```python
from build123d import *

# Parameters (mm, degrees)
SKETCH1_W               = 44
SKETCH1_H               = 20
SKETCH1_R               = 4
SKETCH1_R_2             = 2.55
BOSS_EXTRUDE1_DEPTH     = 7.5
SKETCH2_R               = 2.55
BOSS_EXTRUDE2_DEPTH     = 2.5
SKETCH3_W               = 44
SKETCH3_H               = 5
BOSS_EXTRUDE3_DEPTH     = 10
CUT_EXTRUDE1_DEPTH      = 53.306787322
CUT_EXTRUDE1_DEPTH_BACK = 5


# Read off the part's stored shape, not the designer's step: Sweep1
with BuildPart() as part:
    # Sketch1 → Boss-Extrude1 (new body)
    # profile 1 of 3: a face of its own
    with BuildSketch(Plane(origin=(0, 0, 0), x_dir=(1, 0, 0), z_dir=(0, 1, 0))):
        with BuildLine():
            Line((0, 14), (-6, 14))
            ThreePointArc((-6, 14), (-3.171572875, 12.828427125), (-2, 10))
            ThreePointArc((-2, 10), (-3.171572875, 7.171572875), (-6, 6))
            Line((-6, 6), (0, 6))
            Line((0, 6), (0, 14))
        make_face()
    # profile 2 of 3: a face of its own
    with BuildSketch(Plane(origin=(0, 0, 0), x_dir=(1, 0, 0), z_dir=(0, 1, 0))):
        with Locations((22, 10)):
            Rectangle(SKETCH1_W, SKETCH1_H)
    # profile 3 of 3: a face of its own
    with BuildSketch(Plane(origin=(0, 0, 0), x_dir=(1, 0, 0), z_dir=(0, 1, 0))):
        with Locations((-6, 10)):
            Circle(SKETCH1_R)
        with Locations(Location((-6, 10, 0), (0, 0, 270))):
            Circle(SKETCH1_R_2, mode=Mode.SUBTRACT)
    extrude(amount=BOSS_EXTRUDE1_DEPTH)

    # Sketch2 → Boss-Extrude2 (add)
    # profile 1 of 4: a face of its own
    with BuildSketch(Plane(origin=(0, 7.5, 0), x_dir=(1, 0, 0), z_dir=(0, 1, 0))):
        with BuildLine():
            Line((-6, 6), (0, 6))
            Line((0, 6), (0, 14))
            Line((0, 14), (-6, 14))
            ThreePointArc((-6, 14), (-3.171572875, 12.828427125), (-2, 10))
            ThreePointArc((-2, 10), (-3.171572875, 7.171572875), (-6, 6))
        make_face()
    # profile 2 of 4: a face of its own
    with BuildSketch(Plane(origin=(0, 7.5, 0), x_dir=(1, 0, 0), z_dir=(0, 1, 0))):
        with BuildLine():
            ThreePointArc((-6, 14), (-10, 10), (-6, 6))
            ThreePointArc((-6, 6), (-3.171572875, 7.171572875), (-2, 10))
            ThreePointArc((-2, 10), (-3.171572875, 12.828427125), (-6, 14))
        make_face()
        with Locations(Location((-6, 10, 0), (0, 0, 270))):
            Circle(SKETCH2_R, mode=Mode.SUBTRACT)
    # profile 3 of 4: a face of its own
    with BuildSketch(Plane(origin=(0, 7.5, 0), x_dir=(1, 0, 0), z_dir=(0, 1, 0))):
        with Locations(Location((-6, 10, 0), (0, 0, 270))):
            Circle(SKETCH2_R)
    # profile 4 of 4: a face of its own
    with BuildSketch(Plane(origin=(0, 7.5, 0), x_dir=(1, 0, 0), z_dir=(0, 1, 0))):
        Polygon((0, 0), (44, 0), (44, 20), (0, 20), (0, 14), (0, 6), align=None)
    extrude(amount=BOSS_EXTRUDE2_DEPTH)

    # Sketch3 → Boss-Extrude3 (add)
    with BuildSketch(Plane(origin=(0, 10, 0), x_dir=(1, 0, 0), z_dir=(0, 1, 0))):
        with Locations((22, 2.5)):
            Rectangle(SKETCH3_W, SKETCH3_H)
        with Locations((22, 17.5)):
            Rectangle(SKETCH3_W, SKETCH3_H)
    extrude(amount=BOSS_EXTRUDE3_DEPTH)

    # Sketch4 → Cut-Extrude1 (cut, two sides: drawn at the far end of the back side and taken through both)
    with BuildSketch(Plane(origin=(0, 0, -20), x_dir=(-1, 0, 0), z_dir=(0, 0, -1)).offset(-CUT_EXTRUDE1_DEPTH_BACK)):
        with BuildLine():
            Line((-5, 17.75), (-39, 17.75))
            ThreePointArc((-39, 17.75), (-37.055456352, 16.944543648), (-36.25, 15))
            ThreePointArc((-36.25, 15), (-37.055456352, 13.055456352), (-39, 12.25))
            Line((-39, 12.25), (-5, 12.25))
            ThreePointArc((-5, 12.25), (-7.75, 15), (-5, 17.75))
        make_face()
        with BuildLine():
            ThreePointArc((-36.25, 15), (-37.055456352, 16.944543648), (-39, 17.75))
            Line((-39, 17.75), (-39, 12.25))
            ThreePointArc((-39, 12.25), (-37.055456352, 13.055456352), (-36.25, 15))
        make_face()
        with BuildLine():
            Line((-39, 12.25), (-39, 17.75))
            ThreePointArc((-39, 17.75), (-41.75, 15), (-39, 12.25))
        make_face()
        with BuildLine():
            ThreePointArc((-2.25, 15), (-3.055456352, 16.944543648), (-5, 17.75))
            Line((-5, 17.75), (-5, 12.25))
            ThreePointArc((-5, 12.25), (-3.055456352, 13.055456352), (-2.25, 15))
        make_face()
        with BuildLine():
            Line((-5, 12.25), (-5, 17.75))
            ThreePointArc((-5, 17.75), (-7.75, 15), (-5, 12.25))
        make_face()
    extrude(amount=CUT_EXTRUDE1_DEPTH + CUT_EXTRUDE1_DEPTH_BACK, mode=Mode.SUBTRACT)

    # Sweep1 outline → Sweep1 (revolve)
    with BuildSketch(Plane(origin=(-6, 0, -10), x_dir=(1, 0, 0), z_dir=(0, 0, 1))):
        Polygon((4, 10), (4, 0), (11, 0), (20.5, -5), (38, -5), (38, 0), (20.5, 0), (10.999999705, 10.000000311), align=None)
    revolve(axis=Axis((-6, 0, -10), (0, 1, 0)))


solid = part.part
```
CAD build for the part. Positions are in the model's coordinates, mm. A direction names the side the tool comes from. Round coordinates to 2 decimals unless told otherwise and drop trailing zeros. Write each loop counter-clockwise with the first axis right and the second up, starting at its lowest first coordinate (ties: lowest second). Pieces come first, ordered by that corner, then holes. Notation, with made-up numbers: (72, 76) -> (123, 76) arc R23 ccw to (123, 89) -> close; hole circle Ø8 at (-36, 51.5). An arc over 180 degrees is marked (long way). Answer in a Markdown table with one row per item. Add a question column.
Item 1: Drop flat-ended pins along their axis: pin 1 Ø6 at (x, y) = (15.5, 4) entering from +Z; pin 2 Ø6.5 at (x, z) = (-5.5, -10.5) entering from -Y; pin 3 Ø3 at (x, y) = (15.5, 17) entering from -Z. Give the stop position or say it passes through.
Item 2: Which spindle directions (+Z, -Z, +X, -X, +Y, -Y) get a long thin tool onto all of the face, cutting with end or side? Do faces 4 (the face through (22, 15, -5)), 5 (the face through (-6, 7.5, -10)), 6 (the face through (22, 12.25, -17)), 7 (the face through (22, 20, -18)), 8 (the face through (44, 8, -10)). Say none if no direction does.
Item 3: Saw through at C-C, the plane z = -37.5. Write the cut outline in (x, y).
Item 4: Drill centre lines: line 1 (Z direction, x = 4, y = 11.75); line 2 (Y direction, x = -5, z = -35). Where is each one in solid material? Low to high. Write a range as from..to.
Item 5: Saw through at B-B, the plane y = 1. Write the cut outline in (x, z).
Item 6: Mould opens along X. For faces 1 (the face through (22, 10, -20)), 2 (the face through (41.75, 15.06, -17.46)), 3 (the face through (30.245, -2.465, -21.414)) say: pulls with the +X half, pulls with the -X half, needs draft (parallel to the pull), parting line crosses it, or undercut.
Item 7: Saw through at A-A, the plane x = 29.5. Write the cut outline in (y, z).
Item 8: Saw through at D-D, the plane x = -36.5. Write the cut outline in (y, z).
Findings below:
| question | item | result |
|---|---|---|
| 1 | pin 1 | stops at z = 0 |
| 1 | pin 2 | stops at y = 0 |
| 1 | pin 3 | stops at z = -20 |
| 2 | face 4 | +X, -X, +Y |
| 2 | face 5 | -Y |
| 2 | face 6 | -Z |
| 2 | face 7 | +Z, -Z, +X, -X, +Y |
| 2 | face 8 | +Z, -Z, +X, +Y, -Y |
| 3 | outline | (-32.22, -5) -> (20.22, -5) -> (20.22, 0) -> (-32.22, 0) -> close |
| 4 | line 1 | z = -20..-15, -5..0 |
| 4 | line 2 | y = -5..0 |
| 5 | outline | (10.8, -20) -> (44, -20) -> (44, 0) -> (10.8, 0) arc R19.55 ccw (long way) to start; hole circle Ø5.1 at (-6, -10) |
| 6 | face 1 | needs draft |
| 6 | face 2 | undercut |
| 6 | face 3 | parting line crosses it |
| 7 | outline | (-5, -23.56) -> (0, -23.56) -> (0, -20) -> (12.25, -20) -> (12.25, -15) -> (10, -15) -> (10, -5) -> (20, -5) -> (20, 0) -> (0, 0) -> (0, 3.56) -> (-5, 3.56) -> close; (17.75, -20) -> (20, -20) -> (20, -15) -> (17.75, -15) -> close |
| 8 | outline | (-5, -32.67) -> (0, -32.67) -> (0, 12.67) -> (-5, 12.67) -> close |
